```python
from build123d import *

# Parameters (mm, degrees)
SKETCH1_W           = 560
SKETCH1_H           = 360
SKETCH1_W_2         = 500
SKETCH1_H_2         = 300
EXTRUDE_THIN1_DEPTH = 30
SKETCH2_R           = 7.5
CUT_EXTRUDE1_DEPTH  = 361
EXTRUDE_THIN2_DEPTH = 20
SKETCH4_R           = 10
CUT_EXTRUDE2_DEPTH  = 361


with BuildPart() as part:
    # Sketch1 → Extrude-Thin1 (new body)
    with BuildSketch(Plane(origin=(0, 0, 0), x_dir=(1, 0, 0), z_dir=(0, 1, 0))):
        Rectangle(SKETCH1_W, SKETCH1_H)
        Rectangle(SKETCH1_W_2, SKETCH1_H_2, mode=Mode.SUBTRACT)
    extrude(amount=EXTRUDE_THIN1_DEPTH)

    # Sketch2 → Cut-Extrude1 (cut, through all)
    with BuildSketch(Plane.XY.offset(180)):
        with Locations((-180, 15)):
            Circle(SKETCH2_R)
        with Locations((180, 15)):
            Circle(SKETCH2_R)
    extrude(amount=-CUT_EXTRUDE1_DEPTH, mode=Mode.SUBTRACT)

    # Sketch3 → Extrude-Thin2 (add)
    with BuildSketch(Plane.XY.offset(180)):
        Polygon((-100, 0), (-30, 340), (30, 340), (100, 0), (129.383711298, 6.04958762), (54.452744043, 370), (-54.452744043, 370), (-129.383711298, 6.04958762), align=None)
    extrude_thin2 = extrude(amount=-EXTRUDE_THIN2_DEPTH)

    # Sketch4 → Cut-Extrude2 (cut, through all)
    with BuildSketch(Plane.XY.offset(180)):
        with Locations((0, 355)):
            Circle(SKETCH4_R)
    cut_extrude2 = extrude(amount=-CUT_EXTRUDE2_DEPTH, mode=Mode.SUBTRACT)

    # Mirror1: Extrude-Thin2, Cut-Extrude2 across plane
    add(extrude_thin2.mirror(Plane.XY))
    add(cut_extrude2.mirror(Plane.XY), mode=Mode.SUBTRACT)


solid = part.part
```
Build history of the part. All positions in model axes, mm. A direction names the side the tool comes from. Give positions to 0.01 mm unless a question says otherwise; leave off trailing zeros. Order: outer loops, then holes, each group sorted by start corner. A loop starts at its lowest first (then second) coordinate and runs counter-clockwise, first axis right, second up. Notation, with made-up numbers: M 34.25,60.5 L 56.25,60.5 A27 ccw 56.25,79.5 Z; hole C 26,35.25 d3. An arc over 180 degrees is marked long. Return JSON: item names as keys, results as strings.
Q1. Band-saw the part on B-B (x = 180). Give the cut face in (y, z), then the cut area to 3 significant figures.
Answer list:
{"outline": "M 0,-180 L 7.5,-180 L 7.5,-150 L 0,-150 Z; M 0,150 L 7.5,150 L 7.5,180 L 0,180 Z; M 22.5,-180 L 30,-180 L 30,-150 L 22.5,-150 Z; M 22.5,150 L 30,150 L 30,180 L 22.5,180 Z", "area": "900 mm^2"}
Q2. Wall check: probe 1 along Y at (x, z) = (0, -166.5); probe 2 along Y at (x, z) = (-180, 167); probe 3 along Z at (x, y) = (129, 16). Give the ranges that are in metal, low to high. Write a range as from..to.
Answer list:
{"probe 1": "y = 0..30, 340..345, 365..370", "probe 2": "y = 0..7.5, 22.5..30", "probe 3": "z = -180..-150, 150..180"}
Q3. Band-saw the part on D-D (x = 0). Give the cut face in (y, z), then the cut area to 3 significant figures.
Answer list:
{"outline": "M 0,-180 L 30,-180 L 30,-150 L 0,-150 Z; M 0,150 L 30,150 L 30,180 L 0,180 Z; M 340,-180 L 345,-180 L 345,-160 L 340,-160 Z; M 340,160 L 345,160 L 345,180 L 340,180 Z; M 365,-180 L 370,-180 L 370,-160 L 365,-160 Z; M 365,160 L 370,160 L 370,180 L 365,180 Z", "area": "2,200 mm^2"}
Q4. Band-saw the part on A-A (y = 15). Give the cut face in (x, z).
Answer list:
{"outline": "M -280,-180 L -187.5,-180 L -187.5,-150 L -250,-150 L -250,150 L -187.5,150 L -187.5,180 L -280,180 Z; M -172.5,-180 L 172.5,-180 L 172.5,-150 L -172.5,-150 Z; M -172.5,150 L 172.5,150 L 172.5,180 L -172.5,180 Z; M 187.5,-180 L 280,-180 L 280,180 L 187.5,180 L 187.5,150 L 250,150 L 250,-150 L 187.5,-150 Z"}
Q5. Two-plate mould, pull along X, no slides. Class faces 4 (the face through (0, 340, -170)), 5 (the face through (-88.963, 202.38, -170.14)), 6 (the face through (-56, 226, 160)): pulls with the +X half, pulls with the -X half, needs draft (parallel to the pull), parting line crosses it, or undercut.
Answer list:
{"face 4": "undercut", "face 5": "pulls with the -X half", "face 6": "needs draft"}
Q6. 3-axis set-ups, long thin cutter, end or side, ignore diameter. For faces 1 (the face through (-3, 15, 150)), 2 (the face through (-88.963, 202.38, 170.14)), 3 (the face through (61.465, 187.17, -170.14)): which of +Z, -Z, +X, -X, +Y, -Y reach the whole face in a straight line?
Answer list:
{"face 1": "+Y, -Y", "face 2": "+Z, -Z, -X, +Y", "face 3": "+Z, -Z"}
Q7. Band-saw the part on C-C (z = 116.5). Give the cut face in (x, y).
Answer list:
{"outline": "M -280,0 L -250,0 L -250,30 L -280,30 Z; M 250,0 L 280,0 L 280,30 L 250,30 Z"}
